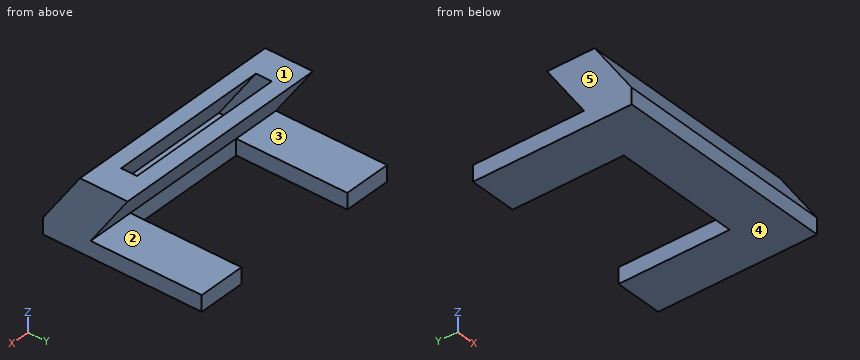
```python
from build123d import *

# Parameters (mm, degrees)
F1_DEPTH = 5
F3_W     = 70
F3_H     = 15
F3_W_2   = 50.9169398992
F3_H_2   = 5


with BuildPart() as f1:
    # F0 (on Top) → F1 (new body)
    with BuildSketch(Plane.XY):
        Polygon((-3.7761517194, 36.0778824546), (-3.7761517194, -13.9221175454), (66.2238482806, -13.9221175454), (66.2238482806, 36.0778824546), (51.2238482806, 36.0778824546), (51.2238482806, 1.0778824546), (11.2238482806, 1.0778824546), (11.2238482806, 36.0778824546), align=None)
    extrude(amount=F1_DEPTH)

    # F4: sweep along a path in F2
    with BuildLine(Plane(origin=(-3.7761517194, 0, 0), x_dir=(0, -1, 0), z_dir=(-1, 0, 0))) as f4_path:
        Line((13.9221175454, 5), (2.2568308138, 22.1641566604))
    # F3 (on face) → F4 (sweep)
    with BuildSketch(Plane.XY.offset(5)):
        with Locations((31.2238482806, -6.4221175454)):
            Rectangle(F3_W, F3_H)
        with Locations((31.2238482806, -6.4221175454)):
            Rectangle(F3_W_2, F3_H_2, mode=Mode.SUBTRACT)
    sweep(path=f4_path.line)


solid = f1.part
```
Read the model definition and answer for the solid it produces. Units are mm, in the model's axes. Face numbers are marked on the shaded views. A direction names the side the tool comes from. Coordinates: 2 decimals unless noted, no trailing zeros. Write each loop counter-clockwise with the first axis right and the second up, starting at its lowest first coordinate (ties: lowest second). Pieces come first, ordered by that corner, then holes. Notation, with made-up numbers: (8, -37) - (45, -37) arc R27 cw to (45, -14) - close; hole circle Ø2 at (45.25, -1). An arc over 180 degrees is marked (long way). Answer as a JSON object with one key per item and string values. Group by question number.
1. Consider L1, parallel to X at y = 28, z = 2.5; L2, parallel to Z at x = 56.5, y = 30; L3, parallel to Y at x = 50, z = 6. Determine where each line is inside the solid, lowest interval first. Write a range as [from, to].
2. Each of these flat-tipped pins is pushed along its axis until it touches: P1, Ø1.5, axis at x = 40, z = 1.5, coming from the +Y side; P2, Ø16.5, axis at x = 58, y = 25, coming from the +Z side; P3, Ø6, axis at x = 18, y = 14.5, coming from the -Z side (3 decimals). Where does it stop, or does it pass through?
3. Which of the six approach directions +Z, -Z, +X, -X, +Y, -Y give full straight-line access (tool end or side, diameter ignored) to the marked faces 1 and 2?
4. The mould has two halves that part along Z. Classify the marked faces 3, 4 and 5: +Z half, -Z half, draft (parallel to the pull), parting line (faces both ways), or undercut.
5. A cutting plane is placed at D-D (z = 7.25). Determine the outline of the cut face in (x, y).
6. A cutting plane is placed at B-B (y = 27). Determine the outline of the cut face in (x, z), plus the area to 3 significant figures.
7. A cutting plane is placed at C-C (y = 6). Determine the outline of the cut face in (x, z), plus the area to 3 significant figures.
8. A cutting plane is placed at A-A (x = 53). Determine the outline of the cut face in (y, z).
Worked out:
{
 "1": {"L1": "x = [-3.78, 11.22], [51.22, 66.22]", "L2": "z = [0, 5]", "L3": "y = [-13.24, -8.24], [-3.24, 1.76]"},
 "2": {"P1": "stops at y = 1.08", "P2": "stops at z = 5", "P3": "stops at z = 20.335"},
 "3": {"face 1": "+Z, +X, -X, +Y, -Y", "face 2": "+X, -X, +Y"},
 "4": {"face 3": "undercut", "face 4": "-Z half", "face 5": "draft"},
 "5": {"outline": "(-3.78, -12.39) - (66.22, -12.39) - (66.22, 2.61) - (-3.78, 2.61) - close; hole (5.77, -7.39) - (56.68, -7.39) - (56.68, -2.39) - (5.77, -2.39) - close"},
 "6": {"outline": "(-3.78, 0) - (11.22, 0) - (11.22, 5) - (-3.78, 5) - close; (51.22, 0) - (66.22, 0) - (66.22, 5) - (51.22, 5) - close", "area": "150 mm²"},
 "7": {"outline": "(-3.78, 0) - (11.22, 0) - (11.22, 5) - (-3.78, 5) - close; (-3.78, 12.24) - (66.22, 12.24) - (66.22, 22.16) - (56.68, 22.16) - (56.68, 19.6) - (5.77, 19.6) - (5.77, 22.16) - (-3.78, 22.16) - close; (51.22, 0) - (66.22, 0) - (66.22, 5) - (51.22, 5) - close", "area": "714 mm²"},
 "8": {"outline": "(-13.92, 0) - (36.08, 0) - (36.08, 5) - (1.08, 5) - (12.74, 22.16) - (7.74, 22.16) - (-3.92, 5) - (-8.92, 5) - (2.74, 22.16) - (-2.26, 22.16) - (-13.92, 5) - close"}
}
